from build123d import *

# Parameters (mm, degrees)
SKETCH1_R               = 5.5245
BOSS_EXTRUDE1_DEPTH     = 40.894
SKETCH2_R               = 1.905
SKETCH2_R_2             = 1.63195
CUT_EXTRUDE1_DEPTH      = 6.5245
CUT_EXTRUDE1_DEPTH_BACK = 6.5245
FILLET1_R               = 0.762


with BuildPart() as part:
    # Sketch1 → Boss-Extrude1 (new body)
    with BuildSketch(Plane(origin=(0, 0, 0), x_dir=(1, 0, 0), z_dir=(0, 1, 0))):
        Circle(SKETCH1_R)
    extrude(amount=BOSS_EXTRUDE1_DEPTH)

    # Sketch2 → Cut-Extrude1 (cut, two sides)
    with BuildSketch(Plane.XY) as cut_extrude1_sk:
        with Locations((0, 28.194)):
            Circle(SKETCH2_R)
        with Locations((0, 6.35)):
            Circle(SKETCH2_R_2)
    extrude(amount=CUT_EXTRUDE1_DEPTH, mode=Mode.SUBTRACT)
    extrude(cut_extrude1_sk.sketch, amount=-CUT_EXTRUDE1_DEPTH_BACK, mode=Mode.SUBTRACT)

    # Fillet1
    fillet1_edges = [part.edges().sort_by_distance(p)[0] for p in [
        (-5.5245, 40.894, 0),
    ]]
    fillet(fillet1_edges, radius=FILLET1_R)


solid = part.part
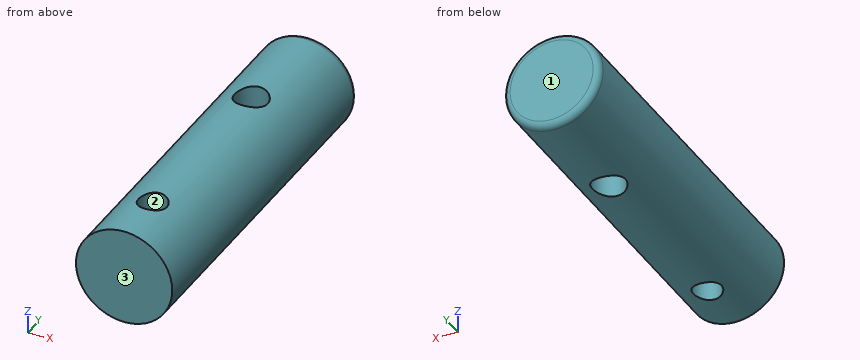
Check sheet for the modelled part. Datum: model origin and axes. Units: mm. Face numbers are marked on the shaded views. Coordinates: 2 decimals unless noted, no trailing zeros. Loops run counter-clockwise (first coordinate to the right, second up) from the corner with the lowest first, then second, coordinate; pieces in that order, holes last. Notation, with made-up numbers: (-9, 58) -> (15, 58) arc R15 cw to (15, 62) -> close; hole circle Ø8 at (7.25, 7.25). An arc over 180 degrees is marked (long way). Write item = value, one per line. Start each with the question number.
1. Section check D-D on y = 7.5. Record the cut outline in (x, z), then the cut area to 3 significant figures.
2. Draft check along Y on the marked faces 1, 2 and 3. Enter one of: released by +Y, released by -Y, zero draft, split by the parting line, or undercut.
3. Section check C-C on y = 21.5. Record the cut outline in (x, z), then the cut area to 3 significant figures.
4. Material ranges on line 1 (Y direction, x = 0, z = -2.75); line 2 (Y direction, x = 1.25, z = 2.5); line 3 (Z direction, x = -0.25, y = 3), recorded low to high.
5. Section check B-B on z = 0. Give the number of separate pieces and of enclosed holes in the cut face, then the cut area to 3 significant figures.
6. Depth check by flat-ended pin: P1, Ø1.5, axis at y = 14, z = -4, coming from the +X side; P2, Ø3, axis at y = 33, z = 4, coming from the -X side. Enter the tip coordinate at first touch or a pass-through.
7. Section check A-A on x = 0. Record the cut outline in (y, z).
Responses:
q1.outline = (-1.16, -5.4) -> (-1.16, 5.4) arc R5.52 ccw to start; (1.16, -5.4) arc R5.52 ccw to (1.16, 5.4) -> close
q1.area = 70.5 mm2
q2.face_1 = released by +Y
q2.face_2 = undercut
q2.face_3 = released by -Y
q3.outline = circle Ø11.05 at (0, 0)
q3.area = 95.9 mm2
q4.line_1 = 0 to 4.72, 7.98 to 26.29, 30.1 to 40.89
q4.line_2 = 0 to 5.3, 7.4 to 26.76, 29.63 to 40.89
q4.line_3 = -5.52 to 5.52
q5.separate_pieces = 1
q5.enclosed_holes = 2
q5.area = 432 mm2
q6.P1 = 4.47
q6.P2 = -4.93
q7.outline = (0, -5.52) -> (4.72, -5.52) -> (4.72, 5.52) -> (0, 5.52) -> close; (7.98, -5.52) -> (26.29, -5.52) -> (26.29, 5.52) -> (7.98, 5.52) -> close; (30.1, -5.52) -> (40.13, -5.52) arc R0.76 ccw to (40.89, -4.76) -> (40.89, 4.76) arc R0.76 ccw to (40.13, 5.52) -> (30.1, 5.52) -> close
